```python
from build123d import *

# Parameters (mm, degrees)
SKETCH1_W           = 200
SKETCH1_H           = 200
BOSS_EXTRUDE1_DEPTH = 5
BOSS_EXTRUDE2_DEPTH = 200
CUT_EXTRUDE9_START  = -200
SKETCH13_W          = 21.4
SKETCH13_H          = 7.5
CUT_EXTRUDE9_DEPTH  = 200
CUT_EXTRUDE14_START = -2
CUT_EXTRUDE14_DEPTH = 3.6
SKETCH17_R          = 2.1
CUT_EXTRUDE15_DEPTH = 16


with BuildPart() as part:
    # Sketch1 → Boss-Extrude1 (new body)
    with BuildSketch(Plane(origin=(0, 0, 0), x_dir=(1, 0, 0), z_dir=(0, 1, 0))):
        Rectangle(SKETCH1_W, SKETCH1_H)
    extrude(amount=BOSS_EXTRUDE1_DEPTH)

    # Sketch9 → Boss-Extrude2 (add)
    with BuildSketch(Plane(origin=(100, 0, 0), x_dir=(0, 0, -1), z_dir=(1, 0, 0))):
        Polygon((-100, 5), (-3, 15), (-3, 5), align=None)
        Polygon((3, 5), (100, 5), (3, 15), align=None)
    extrude(amount=-BOSS_EXTRUDE2_DEPTH)

    # Sketch13 → Cut-Extrude9 (cut)
    with BuildSketch(Plane.ZY.offset(100).offset(CUT_EXTRUDE9_START)):
        with Locations((0, 8.75)):
            Rectangle(SKETCH13_W, SKETCH13_H)
    extrude(amount=CUT_EXTRUDE9_DEPTH, mode=Mode.SUBTRACT)

    # Sketch18 → Cut-Extrude14 (cut)
    with BuildSketch(Plane.XZ.offset(CUT_EXTRUDE14_START)):
        Polygon((-52.136195996, 46.3), (-47.863804004, 46.3), (-45.727608008, 50), (-47.863804004, 53.7), (-52.136195996, 53.7), (-54.272391992, 53.7), (-54.272391992, 46.3), align=None)
        Polygon((47.863804004, 46.3), (52.136195996, 46.3), (54.272391992, 50), (52.136195996, 53.7), (47.863804004, 53.7), (45.727608008, 53.7), (45.727608008, 46.3), align=None)
        Polygon((47.863804004, -53.7), (52.136195996, -53.7), (54.272391992, -50), (52.136195996, -46.3), (47.863804004, -46.3), (45.727608008, -46.3), (45.727608008, -53.7), align=None)
        Polygon((-52.136195996, -53.7), (-47.863804004, -53.7), (-45.727608008, -50), (-47.863804004, -46.3), (-52.136195996, -46.3), (-54.272391992, -46.3), (-54.272391992, -53.7), align=None)
    extrude(amount=-CUT_EXTRUDE14_DEPTH, mode=Mode.SUBTRACT)

    # Sketch17 → Cut-Extrude15 (cut, through all)
    with BuildSketch(Plane.XZ):
        with Locations((-50, 50)):
            Circle(SKETCH17_R)
        with Locations((50, 50)):
            Circle(SKETCH17_R)
        with Locations((50, -50)):
            Circle(SKETCH17_R)
        with Locations((-50, -50)):
            Circle(SKETCH17_R)
    extrude(amount=-CUT_EXTRUDE15_DEPTH, mode=Mode.SUBTRACT)


solid = part.part
```
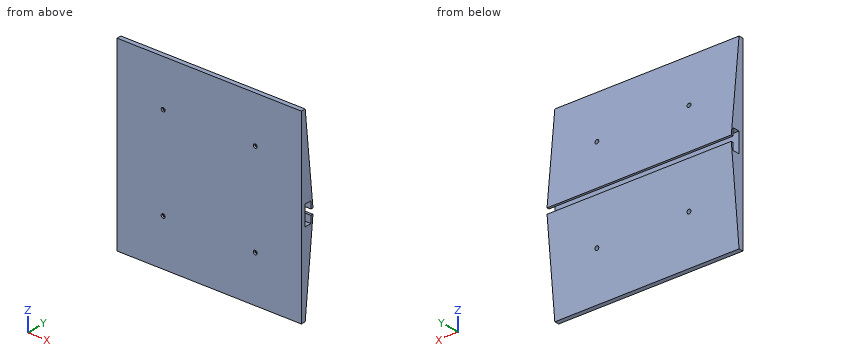
Verification items for the finished model (mm, model axes). Round coordinates to 2 decimals unless told otherwise and drop trailing zeros. Order: outer loops, then holes, each group sorted by start corner. A loop starts at its lowest first (then second) coordinate and runs counter-clockwise, first axis right, second up. Notation, with made-up numbers: (-38, -1) - (5, -1) arc R21 cw to (5, 5) - close; hole circle Ø7 at (9.25, 0). An arc over 180 degrees is marked (long way). Use CSV: the item, a comma, the result in double quotes. Start each with the question number.
1) Go/stop test with flat-tipped pins: P1, Ø5.5, axis at x = -50, z = -50, coming from the +Y side; P2, Ø5, axis at x = -43.5, z = -77.5, coming from the +Y side. Record where each tip stops, or that it passes through.
2) Section check B-B, the plane z = 74. Record the cut outline in (x, y).
3) Thickness scan on L1, parallel to Z at x = -50, y = 0.6; L2, parallel to Y at x = 11, z = -4. Record the ranges inside material, lowest first.
4) Section check A-A, the plane x = -3. Record the cut outline in (y, z).
Answers:
1,P1,"stops at y = 10.44"
1,P2,"stops at y = 7.58"
2,outline,"(-100, 0) - (100, 0) - (100, 7.68) - (-100, 7.68) - close"
3,L1,"z = -100 to -52.1, -47.9 to 47.9, 52.1 to 100"
3,L2,"y = 0 to 5, 12.5 to 14.9"
4,outline,"(0, -100) - (5, -100) - (15, -3) - (12.5, -3) - (12.5, -10.7) - (5, -10.7) - (5, 10.7) - (12.5, 10.7) - (12.5, 3) - (15, 3) - (5, 100) - (0, 100) - close"
